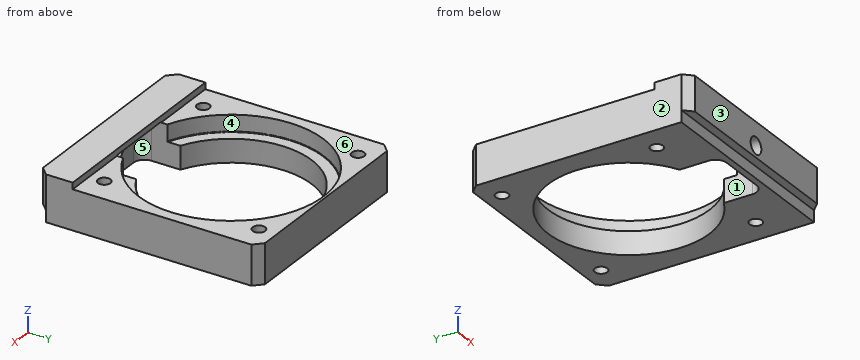
```python
from build123d import *

# Parameters (mm, degrees)
SKETCH1_W                       = 57.15
SKETCH1_H                       = 61.214
BOSS_EXTRUDE1_DEPTH             = 6.35
SKETCH2_W                       = 57.15
SKETCH2_H                       = 51.562
CUT_EXTRUDE1_DEPTH              = 1.778
F_1_1_DIAMETER_HOLE1_D          = 44.45
CUT_EXTRUDE2_DEPTH              = 11.1252
F_14_0_182_DIAMETER_HOLE1_D     = 4.6228
F_14_0_182_DIAMETER_HOLE1_DEPTH = 13.97
F_14_0_182_DIAMETER_HOLE1_TIP   = 1.388829235
SKETCH10_R                      = 25.527
CUT_EXTRUDE3_DEPTH              = 4.572
CHAMFER1_SIZE                   = 2.286
F_8_32_TAPPED_HOLE1_D           = 3.4544
SKETCH13_W                      = 57.15
SKETCH13_H                      = 3.175
CUT_EXTRUDE4_DEPTH              = 2.286
FILLET1_R                       = 0.127


with BuildPart() as part:
    # Sketch1 → Boss-Extrude1 (new body, symmetric)
    with BuildSketch(Plane.XY):
        with Locations((28.575, 30.607)):
            Rectangle(SKETCH1_W, SKETCH1_H)
    extrude(amount=BOSS_EXTRUDE1_DEPTH, both=True)

    # Sketch2 → Cut-Extrude1 (cut)
    with BuildSketch(Plane.XY.offset(6.35)):
        with Locations((28.575, 35.433)):
            Rectangle(SKETCH2_W, SKETCH2_H)
    extrude(amount=-CUT_EXTRUDE1_DEPTH, mode=Mode.SUBTRACT)

    # 1 (1) Diameter Hole1 (through all)
    with Locations(Plane.XY.offset(4.572)):
        with Locations((28.575, 35.052)):
            Hole(F_1_1_DIAMETER_HOLE1_D / 2)

    # Sketch6 → Cut-Extrude2 (cut)
    with BuildSketch(Plane(origin=(0, 0, -6.35), x_dir=(-1, 0, 0), z_dir=(0, 0, -1))):
        with BuildLine():
            Line((-35.052, 3.9624), (-22.098, 3.9624))
            ThreePointArc((-22.098, 3.9624), (-19.942738531, 4.855138531), (-19.05, 7.0104))
            Line((-19.05, 7.0104), (-19.05, 20.953589203))
            Line((-19.05, 20.953589203), (-38.1, 20.953589203))
            Line((-38.1, 20.953589203), (-38.1, 7.0104))
            ThreePointArc((-38.1, 7.0104), (-37.207261469, 4.855138531), (-35.052, 3.9624))
        make_face()
    extrude(amount=-CUT_EXTRUDE2_DEPTH, mode=Mode.SUBTRACT)

    # #14 (0.182) Diameter Hole1
    with Locations(Plane(origin=(0, 3.9624, 0), x_dir=(-1, 0, 0), z_dir=(0, 1, 0))):
        with Locations((-28.575, 0)):
            Hole(F_14_0_182_DIAMETER_HOLE1_D / 2, depth=F_14_0_182_DIAMETER_HOLE1_DEPTH)
            with Locations((0, 0, -(F_14_0_182_DIAMETER_HOLE1_DEPTH + F_14_0_182_DIAMETER_HOLE1_TIP / 2))):  # 118° drill point
                Cone(0, F_14_0_182_DIAMETER_HOLE1_D / 2, F_14_0_182_DIAMETER_HOLE1_TIP, mode=Mode.SUBTRACT)

    # Sketch10 → Cut-Extrude3 (cut)
    with BuildSketch(Plane.XY.offset(4.572)):
        with Locations((28.575, 35.052)):
            Circle(SKETCH10_R)
    extrude(amount=-CUT_EXTRUDE3_DEPTH, mode=Mode.SUBTRACT)

    # Chamfer1
    chamfer1_edges = [part.edges().sort_by_distance(p)[0] for p in [
        (0, 61.214, -0.889),
        (57.15, 61.214, -0.889),
        (57.15, 0, 0),
        (0, 0, 0),
    ]]
    chamfer(chamfer1_edges, length=CHAMFER1_SIZE)

    # #8-32 Tapped Hole1 (through all)
    with Locations(Plane.XY.offset(4.572)):
        with Locations((7.239, 56.388), (49.911, 56.388), (7.239, 13.716), (49.911, 13.716)):
            Hole(F_8_32_TAPPED_HOLE1_D / 2)

    # Sketch13 → Cut-Extrude4 (cut)
    with BuildSketch(Plane.XZ):
        with Locations((28.575, -4.7625)):
            Rectangle(SKETCH13_W, SKETCH13_H)
    extrude(amount=-CUT_EXTRUDE4_DEPTH, mode=Mode.SUBTRACT)

    # Fillet1
    fillet1_edges = [part.edges().sort_by_distance(p)[0] for p in [
        (28.575, 60.579, 0),
    ]]
    fillet(fillet1_edges, radius=FILLET1_R)


solid = part.part
```
Design review of the part built by this model. Coordinates are the model's own, in mm. Face numbers are marked on the shaded views. A direction names the side the tool comes from. Give positions to 0.01 mm unless a question says otherwise; leave off trailing zeros. Write each loop counter-clockwise with the first axis right and the second up, starting at its lowest first coordinate (ties: lowest second). Pieces come first, ordered by that corner, then holes.
(1) Tool access review of the marked faces 4, 5 and 6: name each direction out of +Z, -Z, +X, -X, +Y, -Y from which nothing blocks a thin tool from reaching the whole face with its end or side.
Checked values:
face 4: +Z
face 5: -Z
face 6: +Z, +X, -X, +Y
(2) Add section B-B (z = 1.25). Give the boundary of the cut face in (x, y) (3 decimals).
Checked values:
outline: (0, 2.286) - (2.286, 0) - (26.631, 0) - (26.631, 3.962) - (22.098, 3.962) arc R3.048 cw to (19.05, 7.01) - (19.05, 11.369) arc R25.527 cw (long way) to (38.1, 11.369) - (38.1, 7.01) arc R3.048 cw to (35.052, 3.962) - (30.519, 3.962) - (30.519, 0) - (54.864, 0) - (57.15, 2.286) - (57.15, 58.928) - (54.864, 61.214) - (2.286, 61.214) - (0, 58.928) - close; hole circle Ø3.454 at (7.239, 13.716); hole circle Ø3.454 at (7.239, 56.388); hole circle Ø3.454 at (49.911, 13.716); hole circle Ø3.454 at (49.911, 56.388)
(3) Mouldability with a two-part tool opening along X and no side actions: class the marked faces 1, 2 and 3 as +X half, -X half, draft (parallel to the pull), parting line (faces both ways), or undercut.
Checked values:
face 1: undercut
face 2: -X half
face 3: draft
(4) Clearance check with flat-ended pins moving along their axes: pin 1 Ø5.5 at (x, y) = (49.911, 56.388) entering from +Z; pin 2 Ø1 at (x, z) = (37, -5) entering from -Y; pin 3 Ø0.5 at (x, z) = (33, 5.5) entering from +Y. State where each tip first meets the part, or that it passes through.
Checked values:
pin 1: stops at z = 4.57
pin 2: stops at y = 2.29
pin 3: stops at y = 9.65
(5) Add section A-A (z = -4.75). Give the boundary of the cut face in (x, y) (3 decimals).
Checked values:
outline: (0, 2.286) - (57.15, 2.286) - (57.15, 58.928) - (54.864, 61.214) - (2.286, 61.214) - (0, 58.928) - close; hole circle Ø3.454 at (7.239, 13.716); hole circle Ø3.454 at (7.239, 56.388); hole (19.05, 7.01) arc R3.048 ccw to (22.098, 3.962) - (35.052, 3.962) arc R3.048 ccw to (38.1, 7.01) - (38.1, 14.972) arc R22.225 ccw (long way) to (19.05, 14.972) - close; hole circle Ø3.454 at (49.911, 13.716); hole circle Ø3.454 at (49.911, 56.388)
(6) Add section C-C (z = 5.5). Give the boundary of the cut face in (x, y).
Checked values:
outline: (0, 2.29) - (2.29, 0) - (54.86, 0) - (57.15, 2.29) - (57.15, 9.65) - (0, 9.65) - close
(7) Wall thickness on line 1 along Y through (x, z) = (29, 4); line 2 along X through (y, z) = (35, -2); line 3 along X through (y, z) = (18, -0.25): over which ranges is each line inside the solid? List them lowest first.
Checked values:
line 1: y = 0 to 3.96, 60.58 to 61.21
line 2: x = 0 to 6.35, 50.8 to 57.15
line 3: x = 0 to 14.32, 42.83 to 57.15
